Geometry check sheet. Reference: the model listing, model coordinates, mm. A direction names the side the tool comes from. Coordinates: 2 decimals unless noted, no trailing zeros. Write each loop counter-clockwise with the first axis right and the second up, starting at its lowest first coordinate (ties: lowest second). Pieces come first, ordered by that corner, then holes. Notation, with made-up numbers: (-36.5, 47) -> (-0.5, 47) arc R19 ccw to (-0.5, 54) -> close; hole circle Ø6 at (42, 76). An arc over 180 degrees is marked (long way). Put each result on its own line as item: value. Start each with the question number.
from build123d import *

# Parameters (mm, degrees)
SKETCH1_R                                      = 17.78
BOSS_EXTRUDE1_DEPTH                            = 6.35
CIRPATTERN3_COUNT                              = 3
CUT_EXTRUDE2_REACH                             = 27.934
SKETCH16_R                                     = 7.62
CBORE_FOR_6_SOCKET_HEAD_CAP_SCREW4_D           = 3.6576
CBORE_FOR_6_SOCKET_HEAD_CAP_SCREW4_CBORE_D     = 7.14502
CBORE_FOR_6_SOCKET_HEAD_CAP_SCREW4_CBORE_DEPTH = 3.5052
CIRPATTERN4_COUNT                              = 3


with BuildPart() as part:
    # Sketch1 → Boss-Extrude1 (new body)
    with BuildSketch(Plane(origin=(0, 0, 0), x_dir=(1, 0, 0), z_dir=(0, 1, 0))):
        with Locations(Location((0, 0, 0), (0, 0, 270))):
            Circle(SKETCH1_R)
    extrude(amount=BOSS_EXTRUDE1_DEPTH)

    # Sketch15 → Tap Drill for #8-32 Tap2 (revolve, cut)
    with BuildSketch(Plane(origin=(-8.835910942, 3.105629072, 15.4290336), x_dir=(0.8677746681735182, 0, 0.4969578707258196), z_dir=(0, 1, 0))):
        Polygon((0, 0), (0, 14.149292883), (1.7272, 12.7), (1.7272, 0), align=None)
    tap_drill_for_8_32_tap2 = revolve(axis=Axis((-11.991593421, 3.105629072, 20.939402743), (0.4969578707258196, 0, -0.8677746681735182)), mode=Mode.SUBTRACT)

    # CirPattern3: Tap Drill for #8-32 Tap2 ×3 about axis
    cirpattern3_axis = Axis((0, 6.35, 0), (0, -1, 0))
    for i in range(1, CIRPATTERN3_COUNT):
        add(tap_drill_for_8_32_tap2.rotate(cirpattern3_axis, i * 360 / CIRPATTERN3_COUNT), mode=Mode.SUBTRACT)

    # Sketch16 → Cut-Extrude2 (cut, up to next)
    with BuildSketch(Plane(origin=(0, 6.35, 0), x_dir=(1, 0, 0), z_dir=(0, 1, 0)), mode=Mode.PRIVATE) as cut_extrude2_sk1:
        with Locations(Location((0, 0, 0), (0, 0, 270))):
            Circle(SKETCH16_R)
    cut_extrude2_tool1 = extrude(cut_extrude2_sk1.sketch, amount=-CUT_EXTRUDE2_REACH, mode=Mode.PRIVATE) & part.part
    add(cut_extrude2_tool1.solids().sort_by_distance((0, 6.35, 0))[0], mode=Mode.SUBTRACT)

    # CBORE for #6 Socket Head Cap Screw4 (through all)
    with Locations(Plane(origin=(9.242326206, 0, -7.755232511), x_dir=(0, 0, -1), z_dir=(0, -1, 0))):
        with Locations((0, 0)):
            cbore_for_6_socket_head_cap_screw4 = CounterBoreHole(CBORE_FOR_6_SOCKET_HEAD_CAP_SCREW4_D / 2, CBORE_FOR_6_SOCKET_HEAD_CAP_SCREW4_CBORE_D / 2, CBORE_FOR_6_SOCKET_HEAD_CAP_SCREW4_CBORE_DEPTH)

    # CirPattern4: CBORE for #6 Socket Head Cap Screw4 ×3 about axis
    cirpattern4_axis = Axis((0, 0, 0), (0, 1, 0))
    for i in range(1, CIRPATTERN4_COUNT):
        add(cbore_for_6_socket_head_cap_screw4.rotate(cirpattern4_axis, i * 360 / CIRPATTERN4_COUNT), mode=Mode.SUBTRACT)


solid = part.part
Item 1: Go/stop test with flat-tipped pins: P1, Ø6, axis at x = -11.34, z = -4.13, coming from the -Y side; P2, Ø3, axis at y = 1, z = -6, coming from the -X side; P3, Ø2, axis at y = 3, z = -10, coming from the -X side. Record where each tip stops, or that it passes through.
Item 2: Mould release check, pull along Z, two halves, no side actions. Record for faces 3 (the cylindrical face through (10.48, 4.95, -9.1)), 4 (the cylindrical face through (-17.36, 3.13, -3.85)), 5 (the flat face through (0, 6.35, 8)): released by +Z, released by -Z, zero draft, split by the parting line, or undercut.
Item 3: Section check B-B, the plane x = -6. Give the number of separate pieces and of enclosed holes in the cut face, and give its area (3 significant figures).
Item 4: Section check A-A, the plane z = 3.5. Enter the section's corners in (x, y), and give its area (3 significant figures).
Item 5: Access from +Z, -Z, +X, -X, +Y, -Y to the whole of each face (thin tool, end or side, straight path). Record for faces 1 (the cylindrical face through (-7.795, 1.728, -3.661)), 2 (the cylindrical face through (1.39, 4.95, 13.57)).
Item 6: Scan lines: line 1 along Z through (x, y) = (3, 2.25); line 2 along X through (y, z) = (4.25, 12); line 3 along Z through (x, y) = (6, 2). Record each from-to range of solid material in increasing order. Write a range as [from, to].
From the geometry:
1. P1: y = 3.51
1. P2: x = -17.2
1. P3: x = -15.33
2. face 3: undercut
2. face 4: split by the parting line
2. face 5: zero draft
3. separate pieces: 2
3. enclosed holes: 2
3. area: 115 mm²
4. outline: (-17.43, 0) -> (-6.77, 0) -> (-6.77, 6.35) -> (-17.43, 6.35) -> close; (6.77, 0) -> (17.43, 0) -> (17.43, 6.35) -> (6.77, 6.35) -> close
4. area: 135 mm²
5. face 1: -Y
5. face 2: +Y, -Y
6. line 1: [-17.53, -7], [7, 8.43], [15.34, 17.53]
6. line 2: [-13.12, -8.36], [-5.38, 0.27], [3.92, 13.12]
6. line 3: [-16.74, -9.26], [-6.26, -4.7], [4.7, 16.74]
